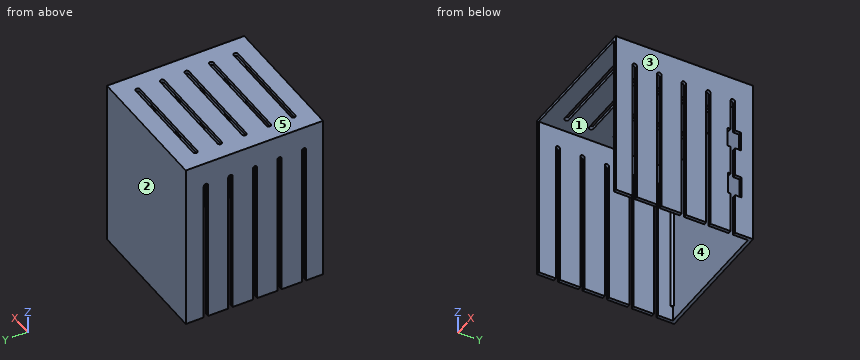
```python
from build123d import *

# Parameters (mm, degrees)
PAD004_DEPTH           = 153
PAD005_DEPTH           = 139
SKETCH007_W            = 124.6
SKETCH007_H            = 126
PAD006_DEPTH           = 3
POCKET002_DEPTH        = 124.601
LINEARPATTERN001_COUNT = 5
LINEARPATTERN001_PITCH = 22.5
POCKET003_DEPTH        = 4
LINEARPATTERN002_COUNT = 5
LINEARPATTERN002_PITCH = 22.5
SKETCH015_R            = 2
POCKET006_DEPTH        = 5
SKETCH016_W            = 12.294895
SKETCH016_H            = 20.342453
SKETCH016_W_2          = 12.071362
SKETCH016_H_2          = 18.107025
POCKET008_DEPTH        = 5


with BuildPart() as part:
    # Sketch006 → Pad004 (new body)
    with BuildSketch(Plane.XY):
        Polygon((62.3, 64.5), (-62.3, 64.5), (-62.3, -61.5), (-59.3, -61.5), (-59.3, 61.5), (59.3, 61.5), (59.3, -61.5), (62.3, -61.5), align=None)
    extrude(amount=PAD004_DEPTH)

    # Sketch008 (on DatumPlane) → Pad005 (join)
    with BuildSketch(Plane.XY.offset(153)):
        Polygon((-59.3, 59.5), (-57.299999, 61.5), (-59.3, 61.5), align=None)
    pad005 = extrude(amount=-PAD005_DEPTH)

    # Mirrored001: Pad005 across Sketch008 V_Axis
    add(pad005.mirror(Plane(origin=(0, 0, 153), x_dir=(0, 0, 1), z_dir=(1, 0, 0))))

    # Sketch007 (on DatumPlane) → Pad006 (join)
    with BuildSketch(Plane.XY.offset(153)):
        with Locations((0, 1.5)):
            Rectangle(SKETCH007_W, SKETCH007_H)
    extrude(amount=PAD006_DEPTH)

    # Sketch010 (on DatumPlane) → Pocket002 (cut, through all)
    with BuildSketch(Plane.YZ.offset(62.3)):
        with BuildLine():
            Line((-46, -89.527603), (-46, 133))
            ThreePointArc((-42, 133), (-44, 135), (-46, 133))
            Line((-42, 133), (-42, -89.527603))
            ThreePointArc((-46, -89.527603), (-44, -91.527603), (-42, -89.527603))
        make_face()
    pocket002 = extrude(amount=-POCKET002_DEPTH, mode=Mode.SUBTRACT)

    # LinearPattern001: Pocket002 ×5
    with Locations(*[(0, i * LINEARPATTERN001_PITCH, 0) for i in range(1, LINEARPATTERN001_COUNT)]):
        add(pocket002, mode=Mode.SUBTRACT)

    # Sketch011 (on Face13 of Pad006) → Pocket003 (cut)
    with BuildSketch(Plane.XY.offset(156)):
        with BuildLine():
            Line((-45.3, -42), (45.3, -42))
            ThreePointArc((45.3, -46), (47.3, -44), (45.3, -42))
            Line((45.3, -46), (-45.3, -46))
            ThreePointArc((-45.3, -42), (-47.3, -44), (-45.3, -46))
        make_face()
    pocket003 = extrude(amount=-POCKET003_DEPTH, mode=Mode.SUBTRACT)

    # LinearPattern002: Pocket003 ×5
    with Locations(*[(0, i * LINEARPATTERN002_PITCH, 0) for i in range(1, LINEARPATTERN002_COUNT)]):
        add(pocket003, mode=Mode.SUBTRACT)

    # Sketch015 (on DatumPlane) → Pocket006 (cut)
    with BuildSketch(Plane.XZ.offset(-64.5)):
        with Locations((-45.035357, 71.063824)):
            Circle(SKETCH015_R)
    extrude(amount=-POCKET006_DEPTH, mode=Mode.SUBTRACT)

    # Sketch016 (on DatumPlane) → Pocket008 (cut)
    with BuildSketch(Plane.YZ.offset(62.3)):
        with Locations((47.763846, 48.412672)):
            Rectangle(SKETCH016_W, SKETCH016_H)
        with Locations((47.204977, 94.909735)):
            Rectangle(SKETCH016_W_2, SKETCH016_H_2)
    extrude(amount=-POCKET008_DEPTH, mode=Mode.SUBTRACT)


with BuildPart() as part_1:
    # Body001 placement: moved
    add(part.part.moved(Location((1.4, 0, 110.1))))


solid = part_1.part
```
CAD build for the part. Positions are in the model's coordinates, mm. Face numbers are marked on the shaded views. A direction names the side the tool comes from. Coordinates: 2 decimals unless noted, no trailing zeros. Write each loop counter-clockwise with the first axis right and the second up, starting at its lowest first coordinate (ties: lowest second). Pieces come first, ordered by that corner, then holes.
(1) Cut at C-C, the plane z = 202. Count the separate pieces of the cut face and the enclosed holes in it, and give its area (3 significant figures).
(2) Cut at B-B, the plane y = 1. List the corners of the cut face in (x, z).
(3) Flat gauge pins, fed straight in: pin 1 (6 mm diameter, centred on x = 26.5, z = 142, fed in from -Y); pin 2 (6 mm diameter, centred on x = 44, y = 49, fed in from -Z). Where does each tip first touch, or does it go through?
(4) Drill centre lines: probe 1 along X at (y, z) = (49, 117); probe 2 along Z at (x, y) = (-46.5, 40.5); probe 3 along Y at (x, z) = (58, 254). Where is each one in solid material? Low to high.
(5) Cut at A-A, the plane x = -39. List the corners of the cut face in (y, z).
(6) 3-axis set-ups, long thin cutter, end or side, ignore diameter. For the marked faces 4 and 5: which of +Z, -Z, +X, -X, +Y, -Y reach the whole face in a straight line?
(7) Two-plate mould, pull along X, no slides. Class the marked faces 1, 2 and 3: +X half, -X half, draft (parallel to the pull), parting line (faces both ways), or undercut.
Geometry says:
1. separate pieces: 11
1. enclosed holes: 0
1. area: 972 mm2
2. outline: (-60.9, 245.1) - (-57.9, 245.1) - (-57.9, 263.1) - (-45.9, 263.1) - (-45.9, 266.1) - (-60.9, 266.1) - close; (48.7, 263.1) - (60.7, 263.1) - (60.7, 245.1) - (63.7, 245.1) - (63.7, 266.1) - (48.7, 266.1) - close
3. pin 1: stops at y = 61.5
3. pin 2: stops at z = 263.1
4. probe 1: x = -60.9 to -57.9, 60.7 to 63.7
4. probe 2: z = 263.1 to 266.1
4. probe 3: y = 61.5 to 64.5
5. outline: (-61.5, 263.1) - (-46, 263.1) - (-46, 266.1) - (-61.5, 266.1) - close; (-42, 263.1) - (-23.5, 263.1) - (-23.5, 266.1) - (-42, 266.1) - close; (-19.5, 263.1) - (-1, 263.1) - (-1, 266.1) - (-19.5, 266.1) - close; (3, 263.1) - (21.5, 263.1) - (21.5, 266.1) - (3, 266.1) - close; (25.5, 263.1) - (44, 263.1) - (44, 266.1) - (25.5, 266.1) - close; (48, 263.1) - (61.5, 263.1) - (61.5, 110.1) - (64.5, 110.1) - (64.5, 266.1) - (48, 266.1) - close
6. face 4: -Z, -Y
6. face 5: +Z, +X, -X, +Y, -Y
7. face 1: undercut
7. face 2: draft
7. face 3: +X half
